Could you check a few things on this model? Use its own coordinates, in mm. A direction names the side the tool comes from. Give positions to 0.01 mm unless a question says otherwise; leave off trailing zeros. Write each loop counter-clockwise with the first axis right and the second up, starting at its lowest first coordinate (ties: lowest second). Pieces come first, ordered by that corner, then holes. Notation, with made-up numbers: (-23.75, 62.5) - (-10.75, 62.5) arc R22 ccw to (-10.75, 84.5) - close; hole circle Ø2 at (-19, 19). An arc over 180 degrees is marked (long way). Use one line per item in the form item = value.
```python
from build123d import *

# Parameters (mm, degrees)
SKETCH1_W           = 649.2
SKETCH1_H           = 25.4
BOSS_EXTRUDE3_DEPTH = 25.4
SKETCH15_R          = 4
CUT_EXTRUDE5_DEPTH  = 25.4
SKETCH11_R          = 4
CUT_EXTRUDE7_DEPTH  = 25.4


with BuildPart() as part:
    # Sketch1 → Boss-Extrude3 (new body)
    with BuildSketch(Plane.XY):
        Polygon((25.4, -700), (25.4, -25.4), (0, 0), (0, -700), align=None)
        Polygon((25.4, -25.4), (674.6, -25.4), (700, 0), (0, 0), align=None)
        Polygon((674.6, -25.4), (700, 0), (700, -700), (674.6, -700), align=None)
        with Locations((350, -537.3)):
            Rectangle(SKETCH1_W, SKETCH1_H)
    extrude(amount=-BOSS_EXTRUDE3_DEPTH)

    # Sketch15 → Cut-Extrude5 (cut)
    with BuildSketch(Plane.XY):
        with Locations((12.7, -240)):
            Circle(SKETCH15_R)
        with Locations((12.7, -390)):
            Circle(SKETCH15_R)
    extrude(amount=-CUT_EXTRUDE5_DEPTH, mode=Mode.SUBTRACT)

    # Sketch11 → Cut-Extrude7 (cut)
    with BuildSketch(Plane.XY):
        with Locations((100, -12.7)):
            Circle(SKETCH11_R)
        with Locations((250, -12.7)):
            Circle(SKETCH11_R)
        with Locations((600, -12.7)):
            Circle(SKETCH11_R)
        with Locations((450, -12.7)):
            Circle(SKETCH11_R)
    extrude(amount=-CUT_EXTRUDE7_DEPTH, mode=Mode.SUBTRACT)


solid = part.part
```
1. Which directions (+Z, -Z, +X, -X, +Y, -Y) give clear straight access to the entire face, cutting with the end or side of a thin tool? Please do faces 4 (the face through (348, -530, -25.4)), 5 (the face through (674.6, -626, -13)), 6 (the face through (345, -25.4, -13)).
Response values:
face_4 = -Z, +X, -X, +Y, -Y
face_5 = +Z, -Z, -Y
face_6 = +Z, -Z
2. Imagine slicing it at B-B, the plane x = 378.5. List the corners of the cut face in (y, z) for me.
Response values:
outline = (-550, -25.4) - (-524.6, -25.4) - (-524.6, 0) - (-550, 0) - close; (-25.4, -25.4) - (0, -25.4) - (0, 0) - (-25.4, 0) - close
3. Imagine slicing it at A-A, the plane y = -296. List the corners of the cut face in (x, z) for me, and give its area (3 significant figures).
Response values:
outline = (0, -25.4) - (25.4, -25.4) - (25.4, 0) - (0, 0) - close; (674.6, -25.4) - (700, -25.4) - (700, 0) - (674.6, 0) - close
area = 1,290 mm²
4. If we mould it in two halves opening along Y, with no side actions, what happens to faces 1 (the face through (345, -550, -13)), 2 (the face through (355, 0, -13)), 3 (the face through (674.6, -278, -13))? For each: pulls with the +Y half, pulls with the -Y half, needs draft (parallel to the pull), parting line crosses it, or undercut.
Response values:
face_1 = pulls with the -Y half
face_2 = pulls with the +Y half
face_3 = undercut
5. For pin 1 (1 mm diameter, centred on x = 516, z = -16, fed in from -Y), with a flat end and sliding along its axis, tell me the tip position at first contact or that it passes through.
Response values:
pin_1 = -550
6. Imagine slicing it at C-C, the plane z = -9. List the corners of the cut face in (x, y) for me, and give its area (3 significant figures).
Response values:
outline = (0, -700) - (25.4, -700) - (25.4, -550) - (674.6, -550) - (674.6, -700) - (700, -700) - (700, 0) - (0, 0) - close; hole circle Ø8 at (12.7, -390); hole circle Ø8 at (12.7, -240); hole (25.4, -524.6) - (674.6, -524.6) - (674.6, -25.4) - (25.4, -25.4) - close; hole circle Ø8 at (100, -12.7); hole circle Ø8 at (250, -12.7); hole circle Ø8 at (450, -12.7); hole circle Ø8 at (600, -12.7)
area = 68,200 mm²
7. If I drill on line 1 (X direction, y = -390, z = -16); line 2 (Y direction, x = 250, z = -8); line 3 (Y direction, x = 12.7, z = -18), over which ranges is the centre line in solid material (lowest first)? Write a range as from..to.
Response values:
line_1 = 0..8.7, 16.7..25.4, 674.6..700
line_2 = -550..-524.6, -25.4..-16.7, -8.7..0
line_3 = -700..-394, -386..-244, -236..0
